Build history of the part. All positions in model axes, mm. Face numbers are marked on the shaded views. Round coordinates to 2 decimals unless told otherwise and drop trailing zeros. Write each loop counter-clockwise with the first axis right and the second up, starting at its lowest first coordinate (ties: lowest second). Pieces come first, ordered by that corner, then holes. Notation, with made-up numbers: (-7.75, -13.75) -> (-3.75, -13.75) arc R21 cw to (-3.75, 0.25) -> close; hole circle Ø11 at (6, 77). An arc over 180 degrees is marked (long way). One line per question, with ' | ' between items.
from build123d import *

# Parameters (mm, degrees)
SKETCH_1_W          = 57
SKETCH_1_H          = 57
EXTRUDE_1_DEPTH     = 41
SKETCH_2_R          = 28.5
EXTRUDE_2_DEPTH     = 53
SKETCH_3_R          = 20
EXTRUDE_3_DEPTH     = 2.5
SKETCH_4_R          = 7
EXTRUDE_4_DEPTH     = 31
SKETCH_7_W          = 57
SKETCH_7_H          = 57
SKETCH_7_R          = 2.6
EXTRUDE_5_DEPTH     = 10
SKETCH_8_W          = 5
SKETCH_8_H          = 4
EXTRUDE_6_DEPTH     = 25
SKETCH_9_R          = 2
CUT_EXTRUDE_1_DEPTH = 6


with BuildPart() as part:
    # 草图1 → 凸台-拉伸1 (new body)
    with BuildSketch(Plane.XY):
        Rectangle(SKETCH_1_W, SKETCH_1_H)
    extrude(amount=EXTRUDE_1_DEPTH)

    # 草图2 → 凸台-拉伸2 (add)
    with BuildSketch(Plane.XY.offset(41)):
        Circle(SKETCH_2_R)
    extrude(amount=EXTRUDE_2_DEPTH)

    # 草图3 → 凸台-拉伸3 (add)
    with BuildSketch(Plane.XY.offset(94)):
        Circle(SKETCH_3_R)
    extrude(amount=EXTRUDE_3_DEPTH)

    # 草图4 → 凸台-拉伸4 (add)
    with BuildSketch(Plane.XY.offset(96.5)):
        Circle(SKETCH_4_R)
    extrude(amount=EXTRUDE_4_DEPTH)

    # 草图7 → 凸台-拉伸5 (add)
    with BuildSketch(Plane.XY.offset(94)):
        Rectangle(SKETCH_7_W, SKETCH_7_H)
        with Locations((-23.57, 23.57)):
            Circle(SKETCH_7_R, mode=Mode.SUBTRACT)
        with Locations((23.57, 23.57)):
            Circle(SKETCH_7_R, mode=Mode.SUBTRACT)
        with Locations((23.57, -23.57)):
            Circle(SKETCH_7_R, mode=Mode.SUBTRACT)
        with Locations((-23.57, -23.57)):
            Circle(SKETCH_7_R, mode=Mode.SUBTRACT)
    extrude(amount=-EXTRUDE_5_DEPTH)

    # 草图8 → 凸台-拉伸6 (add)
    with BuildSketch(Plane.XY.offset(125)):
        with Locations((0, 7)):
            Rectangle(SKETCH_8_W, SKETCH_8_H)
    extrude(amount=-EXTRUDE_6_DEPTH)

    # 草图9 → 切除-拉伸1 (cut)
    with BuildSketch(Plane.XY.offset(127.5)):
        Circle(SKETCH_9_R)
    extrude(amount=-CUT_EXTRUDE_1_DEPTH, mode=Mode.SUBTRACT)


solid = part.part
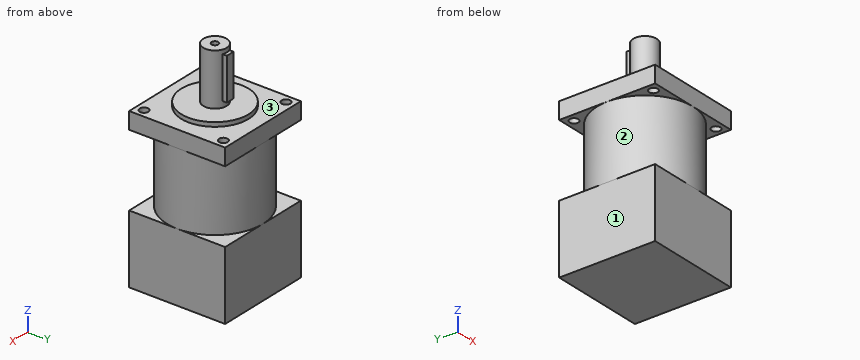
(1) Slice it at C-C (z = 63). Write the cut outline in (x, y).
Calculated:
outline: circle Ø57 at (0, 0)
(2) Drop flat-ended pins along their axis: pin 1 (6 mm diameter, centred on x = 5.5, y = -12.5, fed in from +Z); pin 2 (1 mm diameter, centred on x = 2.5, z = 113.5, fed in from -Y); pin 3 (7 mm diameter, centred on x = 23.57, y = -23.57, fed in from +Z). Give the stop position or say it passes through.
Calculated:
pin 1: z = 96.5 | pin 2: y = -6.71 | pin 3: z = 94
(3) Slice it at D-D (x = 18). Write the cut outline in (y, z), then the cut area to 3 significant figures.
Calculated:
outline: (-28.5, 0) -> (28.5, 0) -> (28.5, 41) -> (22.1, 41) -> (22.1, 84) -> (28.5, 84) -> (28.5, 94) -> (8.72, 94) -> (8.72, 96.5) -> (-8.72, 96.5) -> (-8.72, 94) -> (-28.5, 94) -> (-28.5, 84) -> (-22.1, 84) -> (-22.1, 41) -> (-28.5, 41) -> close | area: 4,850 mm2
(4) Mould opens along Z. For the marked faces 1, 2 and 3 say: pulls with the +Z half, pulls with the -Z half, needs draft (parallel to the pull), parting line crosses it, or undercut.
Calculated:
face 1: needs draft | face 2: undercut | face 3: pulls with the +Z half
(5) Wall check: line 1 (Y direction, x = 0, z = 125.35); line 2 (Y direction, x = 0, z = 123.15); line 3 (Y direction, x = -23, z = 91). Give the ranges that are in metal, low to high. Write a range as from..to.
Calculated:
line 1: -7..-2, 2..7 | line 2: -7..-2, 2..9 | line 3: -28.5..-26.11, -21.03..21.03, 26.11..28.5
(6) Slice it at A-A (x = -23.57). Write the cut outline in (y, z), then the cut area to 3 significant figures.
Calculated:
outline: (-28.5, 0) -> (28.5, 0) -> (28.5, 41) -> (16.02, 41) -> (16.02, 84) -> (20.97, 84) -> (20.97, 94) -> (-20.97, 94) -> (-20.97, 84) -> (-16.02, 84) -> (-16.02, 41) -> (-28.5, 41) -> close; (-28.5, 84) -> (-26.17, 84) -> (-26.17, 94) -> (-28.5, 94) -> close; (26.17, 84) -> (28.5, 84) -> (28.5, 94) -> (26.17, 94) -> close | area: 4,180 mm2
